Autodesk Inventor part; units mm, degrees
ref_plane "body_screw_XY" through (0, -10, 5) normal (0, 0, 1) x (1, 0, 0)
ref_plane "body_screw_YZ" through (0, -10, 5) normal (1, 0, 0) x (0, 1, 0)
ref_plane "body_screw_ZX" through (0, -10, 5) normal (0, 1, 0) x (0, 0, 1)
sketch "Sketch_1" plane through (0, 0, 0) normal (0, 0, 1) x (1, 0, 0)
  line L0 (4, 0) -> (-4, 0)
  line L1 (-4, 14.5) -> (-4, 6.5)
  line L2 (-4, 6.5) -> (-3.5, 6)
  line L3 (-3.5, 6) -> (3.5, 6)
  line L4 (3.5, 6) -> (4, 6.5)
  line L5 (4, 6.5) -> (4, 14.5)
  line L6 (4, 14.5) -> (3.5, 15)
  line L7 (3.5, 15) -> (-3.5, 15)
  line L8 (-3.5, 15) -> (-4, 14.5)
revolve "Revolution1" add sketch "Sketch_1" angle 360 about axis through (4, 0, 0) along (1, 0, 0)
sketch "Sketch_2" plane through (0, 0, 0) normal (1, 0, 0) x (0, 1, 0)
  line L0 (-15, 0.75) -> (-15, -0.75)
  line L1 (-15, -0.75) -> (9.5, -0.75)
  line L2 (9.5, -0.75) -> (9.5, 0.75)
  line L3 (9.5, 0.75) -> (-15, 0.75)
extrude "Extrusion1" cut sketch "Sketch_2" along normal mid plane 8
sketch "Sketch_3" plane through (0, 0, 0) normal (1, 0, 0) x (0, 1, 0)
  line L0 (-10, 15) -> (-10, 0)
  line L1 (-10, 0) -> (-11.7, 0)
  line L2 (-11.7, 0) -> (-11.7, 5)
  line L3 (-11.7, 5) -> (-13, 5)
  line L4 (-13, 5) -> (-13, 15)
  line L5 (-13, 15) -> (-10, 15)
  line L6 (-10, 15) -> (-10, 0)
revolve "Revolution2" cut sketch "Sketch_3" angle 360 about axis through (0, -10, 15) along (0, 0, 1)
sketch "Sketch_4" plane through (0, 0, 0) normal (1, 0, 0) x (0, 1, 0)
  line L0 (-10, -15.75) -> (-10, -0.75)
  line L1 (-10, -0.75) -> (-8.5, -0.75)
  line L2 (-8.5, -0.75) -> (-8.7705, -1.0205)
  line L3 (-8.7705, -1.0205) -> (-8.7705, -15.75)
  line L4 (-8.7705, -15.75) -> (-10, -15.75)
  line L5 (-10, -15.75) -> (-10, -0.75)
revolve "Revolution3" cut sketch "Sketch_4" angle 360 about axis through (0, -10, -15.75) along (0, 0, -1)
thread "Thread1"
sketch "Sketch_7" plane through (0, 0, -11) normal (0, 0, 1) x (1, 0, 0)
  line L0 (4, 0) -> (-4, 0)
  line L1 (-4, 0) -> (-4, 2.5)
  line L2 (-4, 2.5) -> (-3.567, 2.067)
  line L3 (-3.567, 2.067) -> (3.567, 2.067)
  line L4 (3.567, 2.067) -> (4, 2.5)
  line L5 (4, 2.5) -> (4, 0)
  line L6 (4, 0) -> (-4, 0)
revolve "Revolution4" cut sketch "Sketch_7" angle 360 about axis through (4, 0, -11) along (1, 0, 0)
thread "Thread2"
sketch "Sketch_8" plane through (0, 0, 11) normal (0, 0, 1) x (1, 0, 0)
  line L0 (4, 0) -> (-4, 0)
  line L1 (-4, 0) -> (-4, 2.5)
  line L2 (-4, 2.5) -> (-3.567, 2.067)
  line L3 (-3.567, 2.067) -> (3.567, 2.067)
  line L4 (3.567, 2.067) -> (4, 2.5)
  line L5 (4, 2.5) -> (4, 0)
  line L6 (4, 0) -> (-4, 0)
revolve "Revolution5" cut sketch "Sketch_8" angle 360 about axis through (4, 0, 11) along (1, 0, 0)
thread "Thread3"
ref_plane "body_screw_XY" through (0, -10, 5) normal (0, 0, 1) x (1, 0, 0)
ref_plane "body_screw_YZ" through (0, -10, 5) normal (1, 0, 0) x (0, 1, 0)
ref_plane "body_screw_ZX" through (0, -10, 5) normal (0, 1, 0) x (0, 0, 1)
properties part number "SCSW12-8b"
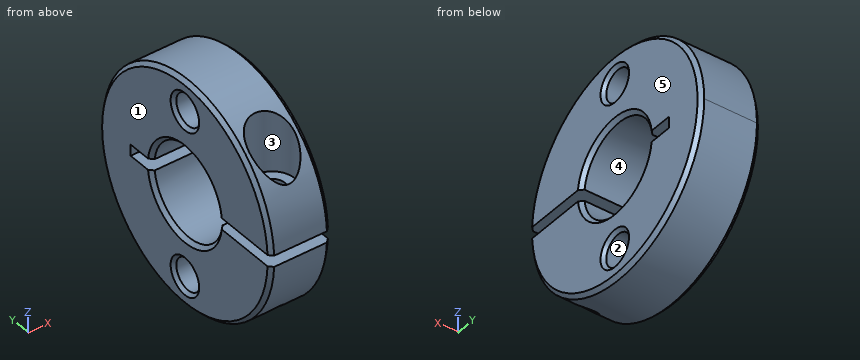
Could you check a few things on this model? Use its own coordinates, in mm. Face numbers are marked on the shaded views. A direction names the side the tool comes from. Round coordinates to 2 decimals unless told otherwise and drop trailing zeros. Write each loop counter-clockwise with the first axis right and the second up, starting at its lowest first coordinate (ties: lowest second). Pieces come first, ordered by that corner, then holes. Notation, with made-up numbers: (-19, 60.5) - (-15, 60.5) arc R33 ccw to (-15, 99.5) - close; hole circle Ø5 at (-40, -21.75). An arc over 180 degrees is marked (long way). Use a Markdown table: item, result.
Q1. I want a section at B-B (x = 0). List the corners of the cut face in (y, z) for me.
Output values:
| item | result |
|---|---|
| outline | (-14.98, -0.75) arc R15 ccw to (-11.23, -9.94) - (-11.23, -1.02) - (-11.5, -0.75) - close; (-14.98, 0.75) - (-11.7, 0.75) - (-11.7, 5) - (-13, 5) - (-13, 7.48) arc R15 ccw to start; (-8.77, -12.17) arc R15 ccw (long way) to (-7, 13.27) - (-7, 5) - (-8.3, 5) - (-8.3, 0.75) - (-5.95, 0.75) arc R6 cw to (5.95, 0.75) - (9.5, 0.75) - (9.5, -0.75) - (5.95, -0.75) arc R6 cw to (-5.95, -0.75) - (-8.5, -0.75) - (-8.77, -1.02) - close; hole circle Ø4.13 at (0, -11); hole circle Ø4.13 at (0, 11) |
Q2. For the marked faces 3, 4 and 5, which set-ups out of +Z, -Z, +X, -X, +Y, -Y let a thin tool reach every point of the face, with its end or its side?
Output values:
| item | result |
|---|---|
| face 3 | +Z |
| face 4 | +X, -X |
| face 5 | +Z, -Z, +X, +Y, -Y |
Q3. I want a section at A-A (y = 0). Count the separate pieces of the cut face and the enclosed holes in it, plus the area to 3 significant figures.
Output values:
| item | result |
|---|---|
| separate pieces | 4 |
| enclosed holes | 0 |
| area | 76.1 mm2 |
Q4. Please list where these lines run through material, in increasing order: L1, parallel to Z at x = -1.5, y = 0; L2, parallel to X at y = -10, z = 6.75; L3, parallel to Y at x = -1, z = 4.
Output values:
| item | result |
|---|---|
| L1 | -15 to -13.07, -8.93 to -6, 6 to 8.93, 13.07 to 15 |
| L2 | -4 to -3, 3 to 4 |
| L3 | -14.46 to -11.37, -8.63 to -4.47, 4.47 to 14.46 |
Q5. For pin 1 (3.5 mm diameter, centred on y = 0, z = 11, fed in from +X); pin 2 (1.8 mm diameter, centred on x = 1.5, y = 8.5, fed in from +Z); pin 3 (1.5 mm diameter, centred on x = 2.5, z = 2.5, fed in from -Y); pin 4 (3 mm diameter, centred on x = -0.5, y = 7, fed in from -Z), each with a flat end and sliding along its axis, tell me the tip position at first contact or that it passes through.
Output values:
| item | result |
|---|---|
| pin 1 | through |
| pin 2 | z = 12.93 |
| pin 3 | y = -14.9 |
| pin 4 | z = -13.96 |
Q6. Thinking about a two-plate mould opening in Y: for the marked faces 1 and 2, which applies, released by +Y, released by -Y, zero draft, split by the parting line, or undercut?
Output values:
| item | result |
|---|---|
| face 1 | zero draft |
| face 2 | undercut |
Q7. I want a section at C-C (x = -2.5). List the corners of the cut face in (y, z) for me, plus the area to 3 significant figures.
Output values:
| item | result |
|---|---|
| outline | (-14.98, -0.75) arc R15 ccw (long way) to (-8.34, 12.47) - (-8.34, 5) - (-11.66, 5) - (-11.66, 9.44) arc R15 ccw to (-14.98, 0.75) - (-5.95, 0.75) arc R6 cw to (5.95, 0.75) - (9.5, 0.75) - (9.5, -0.75) - (5.95, -0.75) arc R6 cw to (-5.95, -0.75) - close; hole circle Ø4.13 at (0, -11); hole circle Ø4.13 at (0, 11) |
| area | 528 mm2 |
